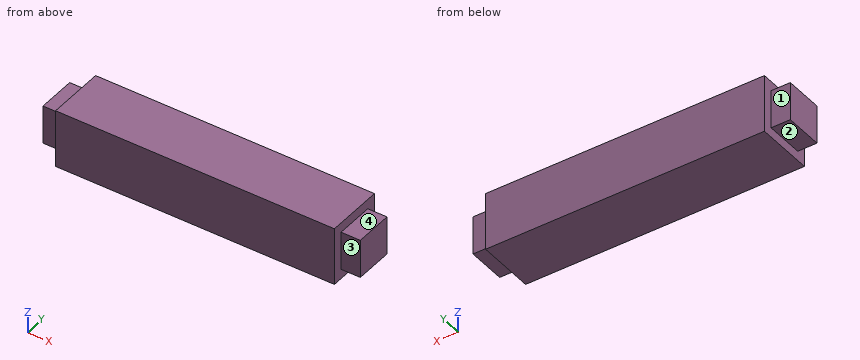
from build123d import *

# Parameters (mm, degrees)
SKETCH1_W           = 145
SKETCH1_H           = 30
BOSS_EXTRUDE1_DEPTH = 15
SKETCH2_W           = 20
SKETCH2_H           = 20
BOSS_EXTRUDE2_DEPTH = 10
SKETCH3_W           = 20
SKETCH3_H           = 20
BOSS_EXTRUDE3_DEPTH = 10


with BuildPart() as part:
    # Sketch1 → Boss-Extrude1 (new, symmetric)
    with BuildSketch(Plane.XY):
        Rectangle(SKETCH1_W, SKETCH1_H)
    extrude(amount=BOSS_EXTRUDE1_DEPTH, both=True)

    # Sketch2 → Boss-Extrude2 (add)
    with BuildSketch(Plane(origin=(72.5, 0, 0), x_dir=(0, 0, -1), z_dir=(1, 0, 0))):
        Rectangle(SKETCH2_W, SKETCH2_H)
    extrude(amount=BOSS_EXTRUDE2_DEPTH)

    # Sketch3 → Boss-Extrude3 (add)
    with BuildSketch(Plane.ZY.offset(72.5)):
        Rectangle(SKETCH3_W, SKETCH3_H)
    extrude(amount=BOSS_EXTRUDE3_DEPTH)


solid = part.part
Build history of the part. All positions in model axes, mm. Face numbers are marked on the shaded views. A direction names the side the tool comes from. Give positions to 0.01 mm unless a question says otherwise; leave off trailing zeros. Order: outer loops, then holes, each group sorted by start corner. A loop starts at its lowest first (then second) coordinate and runs counter-clockwise, first axis right, second up. Notation, with made-up numbers: M -23,-31 L -16,-31 A35 ccw -16,8 Z; hole C -0.75,71 d4. An arc over 180 degrees is marked long. Put each result on its own line as item: value.
Item 1: Flat gauge pins, fed straight in: pin 1 Ø5 at (x, z) = (76.5, -1) entering from +Y; pin 2 Ø5 at (x, y) = (78.5, 1.5) entering from -Z; pin 3 Ø3 at (x, z) = (75.5, -5) entering from -Y; pin 4 Ø8 at (x, y) = (-76, -3.5) entering from -Z. Where does each tip first touch, or does it go through?
From the geometry:
pin 1: stops at y = 10
pin 2: stops at z = -10
pin 3: stops at y = -10
pin 4: stops at z = -15
Item 2: Slice it at A-A, the plane z = 7.5. Write the cut outline in (x, y).
From the geometry:
outline: M -82.5,-10 L -72.5,-10 L -72.5,-15 L 72.5,-15 L 72.5,-10 L 82.5,-10 L 82.5,10 L 72.5,10 L 72.5,15 L -72.5,15 L -72.5,10 L -82.5,10 Z
Item 3: 3-axis set-ups, long thin cutter, end or side, ignore diameter. For the marked faces 1, 2, 3 and 4: which of +Z, -Z, +X, -X, +Y, -Y reach the whole face in a straight line?
From the geometry:
face 1: +Z, -Z, -X, +Y
face 2: -Z, -X, +Y, -Y
face 3: +Z, -Z, +X, -Y
face 4: +Z, +X, +Y, -Y
Item 4: Probe line 1 (X direction, y = 4, z = -10.5). List the from-to ranges inside material, lowest first. Write a range as [from, to].
From the geometry:
line 1: x = [-72.5, 72.5]
